```python
from build123d import *

# Parameters (mm, degrees)
EXTRUDE028_DEPTH = 2
EXTRUDE029_DEPTH = 1
EXTRUDE027_DEPTH = 4


with BuildPart() as hangerlockfront:
    # Sketch037 → Extrude028 (new body)
    with BuildSketch(Plane.XZ):
        with BuildLine():
            ThreePointArc((-7.5, 10), (0, -12.5), (7.5, 10))
            Line((7.5, 10), (7.5, 17.400658))
            Line((6.5, 17.400658), (7.5, 17.400658))
            ThreePointArc((-6.5, 17.400658), (0, 15), (6.5, 17.400658))
            Line((-7.5, 17.400658), (-6.5, 17.400658))
            Line((-7.5, 10), (-7.5, 17.400658))
        make_face()
    extrude(amount=EXTRUDE028_DEPTH)


with BuildPart() as hangerlockfront_1:
    # Extrude028 placement: moved
    add(hangerlockfront.part.moved(Location((0, -5, 0))))


with BuildPart() as hangerlockspacer:
    # Sketch038 → Extrude029 (new body)
    with BuildSketch(Plane.XZ):
        with BuildLine():
            ThreePointArc((-5, 8.660254), (0, -10), (5, 8.660254))
            Line((5, 8.660254), (5, 15.834849))
            Line((4, 15.834849), (5, 15.834849))
            ThreePointArc((-4, 15.834849), (0, 15), (4, 15.834849))
            Line((-5, 15.834849), (-4, 15.834849))
            Line((-5, 8.660254), (-5, 15.834849))
        make_face()
    extrude(amount=EXTRUDE029_DEPTH)


with BuildPart() as hangerlockspacer_1:
    # Extrude029 placement: moved
    add(hangerlockspacer.part.moved(Location((0, -4, 0))))


with BuildPart() as hangerlockright:
    # Sketch036 → Extrude027 (new body)
    with BuildSketch(Plane.XZ):
        with BuildLine():
            ThreePointArc((-5, 8.660254), (0, -10), (5, 8.660254))
            Line((5, 8.660254), (5, 22))
            Line((4, 22), (5, 22))
            ThreePointArc((-4, 22), (0, 20), (4, 22))
            Line((-5, 22), (-4, 22))
            Line((-5, 8.660254), (-5, 22))
        make_face()
    extrude(amount=EXTRUDE027_DEPTH)

    # Fusion002: union HangerLockFront, HangerLockSpacer
    add(hangerlockfront_1.part)
    add(hangerlockspacer_1.part)


with BuildPart() as hangerlockright_1:
    # Fusion002 placement: moved
    add(hangerlockright.part.moved(Location((70, 40, 200))))


solid = hangerlockright_1.part
```
Design review of the part built by this model. Coordinates are the model's own, in mm. A direction names the side the tool comes from. Coordinates: 2 decimals unless noted, no trailing zeros. Loops run counter-clockwise (first coordinate to the right, second up) from the corner with the lowest first, then second, coordinate; pieces in that order, holes last.
Q1. To check wall thickness, follow line 1 (X direction, y = 34, z = 214.5); line 2 (Y direction, x = 81.75, z = 199.5); line 3 (X direction, y = 37.75, z = 219). State the ranges of each line that lie inside material, in increasing order.
Reported:
line 1: x = 62.5 to 77.5
line 2: y = 33 to 35
line 3: x = 65 to 75
Q2. We need section A-A on z = 200. State the section outline as (x, y) points.
Reported:
outline: (57.5, 33) - (82.5, 33) - (82.5, 35) - (80, 35) - (80, 40) - (60, 40) - (60, 35) - (57.5, 35) - close
Q3. We need section B-B on x = 70. State the section outline as (y, z) points.
Reported:
outline: (33, 187.5) - (35, 187.5) - (35, 190) - (40, 190) - (40, 220) - (36, 220) - (36, 215) - (33, 215) - close
Q4. The part is to be moulded in two halves that separate along Y. For faces 1 (the face through (70, 40, 206)), 2 (the face through (65.5, 35.5, 215.835)), 3 (the face through (77, 34, 217.401)), say which applies: +Y half, -Y half, draft (parallel to the pull), parting line (faces both ways), or undercut.
Reported:
face 1: +Y half
face 2: undercut
face 3: draft
Q5. For pin 1 (4 mm diameter, centred on y = 36.5, z = 217.5, fed in from +X); pin 2 (1.6 mm diameter, centred on y = 34.5, z = 213.5, fed in from -X); pin 3 (8 mm diameter, centred on x = 60.5, z = 213.5, fed in from +Y), all flat-tipped, find the tip position at first contact; note any pin that passes through.
Reported:
pin 1: stops at x = 77.5
pin 2: stops at x = 62.5
pin 3: stops at y = 35
Q6. We need section D-D on y = 37.25. State the section outline as (x, z) points, and give its area (3 significant figures).
Reported:
outline: (65, 208.66) arc R10 ccw (long way) to (75, 208.66) - (75, 222) - (74, 222) arc R5 cw to (66, 222) - (65, 222) - close
area: 427 mm2
Q7. Tool access review of faces 4 (the face through (74.5, 35.5, 215.835)), 5 (the face through (70, 38, 190)), 6 (the face through (77.5, 34, 214)): name each direction out of +Z, -Z, +X, -X, +Y, -Y from which nothing blocks a thin tool from reaching the whole face with its end or side.
Reported:
face 4: +Z, +X, -X
face 5: +Y
face 6: +Z, +X, +Y, -Y
Q8. We need section C-C on y = 34. State the section outline as (x, z) points, and give its area (3 significant figures).
Reported:
outline: (62.5, 210) arc R12.5 ccw (long way) to (77.5, 210) - (77.5, 217.4) - (76.5, 217.4) arc R10 cw to (63.5, 217.4) - (62.5, 217.4) - close
area: 555 mm2
